For this review, take the finished solid that the model builds, in its own axes (mm). Face numbers are marked on the shaded views. A direction names the side the tool comes from. Give positions to 0.01 mm unless a question says otherwise; leave off trailing zeros. Order: outer loops, then holes, each group sorted by start corner. A loop starts at its lowest first (then second) coordinate and runs counter-clockwise, first axis right, second up.
Item 1: Machinability: for the marked faces 4, 5, 6, 7 and 8, which of the approach directions +Z, -Z, +X, -X, +Y, -Y give a long, thin tool a straight path to every point of the face, cutting with its end or side? Answer none if there is none.
Item 2: Consider section D-D (x = 148.5). Give the boundary of the cut face in (y, z), plus the area to 3 significant figures.
Item 3: For probe 1 along Z at (x, y) = (47, 217.5); probe 2 along Z at (x, y) = (131.5, 196); probe 3 along X at (y, z) = (115, 149), list the stretches that pass through material, from the lowest coordinate up.
Item 4: Consider section C-C (z = -82). Give the boundary of the cut face in (x, y).
Item 5: For P1, Ø6, axis at x = 66.5, z = 117.5, coming from the -Y side, flat-tipped, find the tip position at first contact; note if it passes through.
Item 6: Consider section A-A (y = 77.5). Give the boundary of the cut face in (x, z).
Item 7: The part is to be moulded in two halves that separate along X. For the marked faces 1, 2 and 3, say which applies: released by +X, released by -X, zero draft, split by the parting line, or undercut.
Item 8: Consider section B-B (x = -129). Give the boundary of the cut face in (y, z).
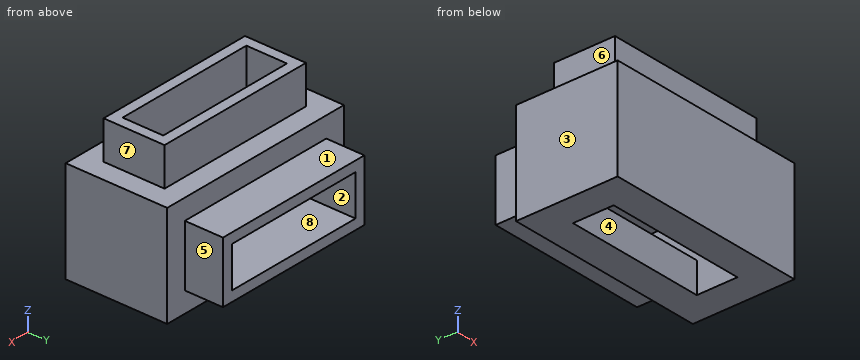
Autodesk Inventor part; units mm, degrees
ref_plane "YZ Plane" through (0, 0, 0) normal (1, 0, 0) x (0, 1, 0)
ref_plane "XZ Plane" through (0, 0, 0) normal (0, 1, 0) x (-1, 0, 0)
ref_plane "XY Plane" through (0, 0, 0) normal (0, 0, 1) x (1, 0, 0)
sketch "Sketch1" plane through (0, 0, 0) normal (0, 1, 0) x (-1, 0, 0)
  line L0 (200, 100) -> (-200, 100)
  line L1 (-200, 100) -> (-200, -100)
  line L2 (-200, -100) -> (200, -100)
  line L3 (200, -100) -> (200, 100)
  line L4 (0, -140) -> (0, 140)
  line L5 (-280, 0) -> (280, 0)
  point P0 (0, 0)
  dimension "d0" = 400
  dimension "d1" = 200
extrude "Extrusion1" add sketch "Sketch1" along normal blind 200
sketch "Sketch2" plane through (-200, 0, 100) normal (0, 0, 1) x (1, 0, 0)
  line L0 (0, 0) -> (400, 0)
  line L1 (400, 0) -> (400, 200)
  line L2 (0, 200) -> (400, 200)
  line L3 (0, 0) -> (0, 200)
  line L4 (360, 160) -> (360, 40)
  line L5 (360, 40) -> (40, 40)
  line L6 (40, 40) -> (40, 160)
  line L7 (40, 160) -> (360, 160)
  point P0 (200, 0)
  dimension "d4" = 40
extrude "Extrusion2" add sketch "Sketch2" along normal blind 75 contours L4 L5 L6 L7
sketch "Sketch3" plane through (-200, 0, 175) normal (0, 0, 1) x (1, 0, 0)
  line L0 (360, 40) -> (360, 160)
  line L1 (360, 160) -> (40, 160)
  line L2 (40, 160) -> (40, 40)
  line L3 (40, 40) -> (360, 40)
  line L4 (60, 140) -> (340, 140)
  line L5 (340, 140) -> (340, 60)
  line L6 (340, 60) -> (60, 60)
  line L7 (60, 60) -> (60, 140)
  point P0 (200, 0)
  dimension "d7" = 20
extrude "Extrusion3" cut sketch "Sketch3" against normal through all contours L4 L5 L6 L7
sketch "Sketch5" plane through (0, 200, 0) normal (0, 1, 0) x (1, 0, 0)
  line L0 (-200, -100) -> (200, -100)
  line L1 (200, -100) -> (200, 100)
  line L2 (200, 100) -> (-200, 100)
  line L3 (-200, 100) -> (-200, -100)
  line L4 (-160, 60) -> (160, 60)
  line L5 (160, 60) -> (160, -60)
  line L6 (160, -60) -> (-160, -60)
  line L7 (-160, -60) -> (-160, 60)
  point P0 (0, 0)
  dimension "d19" = 40
extrude "Extrusion4" add sketch "Sketch5" along normal blind 75 contours L4 L5 L6 L7
sketch "Sketch6" plane through (0, 275, 0) normal (0, 1, 0) x (1, 0, 0)
  line L0 (160, 60) -> (-160, 60)
  line L1 (-160, 60) -> (-160, -60)
  line L2 (-160, -60) -> (160, -60)
  line L3 (160, -60) -> (160, 60)
  line L4 (-140, 40) -> (140, 40)
  line L5 (140, 40) -> (140, -40)
  line L6 (140, -40) -> (-140, -40)
  line L7 (-140, -40) -> (-140, 40)
  point P0 (0, 0)
  dimension "d22" = 20
extrude "Extrusion5" cut sketch "Sketch6" against normal up to surface (135 mm away) contours L4 L5 L6 L7
properties part number "fillet"
Resolved:
1. face 4: +Z, -Z
1. face 5: +Z, -Z, +X, +Y
1. face 6: +Z, -X, +Y, -Y
1. face 7: +Z, +X, +Y, -Y
1. face 8: +Y
2. outline: (0, -100) - (200, -100) - (200, -60) - (275, -60) - (275, 60) - (200, 60) - (200, 100) - (160, 100) - (160, 175) - (40, 175) - (40, 100) - (0, 100) - close
2. area: 58,000 mm2
3. probe 1: z = -60 to -40, 40 to 60
3. probe 2: z = -100 to -40, 40 to 100
3. probe 3: x = -160 to -140, 140 to 160
4. outline: (-200, 0) - (200, 0) - (200, 200) - (-200, 200) - close; hole (-140, 60) - (140, 60) - (140, 140) - (-140, 140) - close
5. P1: stops at y = 40
6. outline: (-200, -100) - (-140, -100) - (-140, 175) - (-160, 175) - (-160, 100) - (-200, 100) - close; (140, -100) - (200, -100) - (200, 100) - (160, 100) - (160, 175) - (140, 175) - close
7. face 1: zero draft
7. face 2: undercut
7. face 3: released by -X
8. outline: (0, -100) - (60, -100) - (60, 175) - (40, 175) - (40, 100) - (0, 100) - close; (140, -100) - (200, -100) - (200, -60) - (275, -60) - (275, -40) - (140, -40) - close; (140, 40) - (275, 40) - (275, 60) - (200, 60) - (200, 100) - (160, 100) - (160, 175) - (140, 175) - close
